from build123d import *

# Parameters (mm, degrees)
SKETCH1_W           = 25
SKETCH1_H           = 40
BOSS_EXTRUDE1_DEPTH = 8
FILLET1_R           = 2
CUT_EXTRUDE1_DEPTH  = 0.1


with BuildPart() as part:
    # Sketch1 → Boss-Extrude1 (new body)
    with BuildSketch(Plane.XY):
        Rectangle(SKETCH1_W, SKETCH1_H)
    extrude(amount=BOSS_EXTRUDE1_DEPTH)

    # Fillet1
    fillet1_edges = [part.edges().sort_by_distance(p)[0] for p in [
        (-12.5, 0, 8),
        (0, -20, 8),
        (12.5, 0, 8),
        (0, -20, 0),
        (-12.5, 0, 0),
        (0, 20, 0),
        (12.5, 0, 0),
        (12.5, -20, 4),
        (-12.5, -20, 4),
        (-12.5, 20, 4),
        (12.5, 20, 4),
        (0, 20, 8),
    ]]
    fillet(fillet1_edges, radius=FILLET1_R)

    # Sketch2 → Cut-Extrude1 (cut)
    with BuildSketch(Plane.XY.offset(8)):
        Polygon((-2.061020471, 8.237438207), (2.736573232, 8.237438207), (-0.031843364, 1.854183508), (2.068180648, 1.854183508), (-2.268382383, -6.039716385), (-0.867604628, 1.003082881), (-3.464302761, 1.003082881), align=None)
    extrude(amount=-CUT_EXTRUDE1_DEPTH, mode=Mode.SUBTRACT)


solid = part.part
Model file for the job. Use its own axes, mm. Round coordinates to 2 decimals unless told otherwise and drop trailing zeros. Loops run counter-clockwise (first coordinate to the right, second up) from the corner with the lowest first, then second, coordinate; pieces in that order, holes last. Notation, with made-up numbers: M 30,69.5 L 86,69.5 A19 cw 86,91.5 Z; hole C -27,-15.75 d1. An arc over 180 degrees is marked long. One line per question, with ' | ' between items.
1) Band-saw the part on A-A (y = 13). Give the cut face in (x, z).
Solved:
outline: M -12.5,2 A2 ccw -10.5,0 L 10.5,0 A2 ccw 12.5,2 L 12.5,6 A2 ccw 10.5,8 L -10.5,8 A2 ccw -12.5,6 Z
2) Drill centre lines: line 1 along Z through (x, y) = (1.25, 1); line 2 along Y through (x, z) = (10.5, 7); line 3 along Y through (x, z) = (6.5, 1.25). Where is each one in solid material? Low to high.
Solved:
line 1: z = 0 to 7.9 | line 2: y = -19.73 to 19.73 | line 3: y = -19.85 to 19.85
3) Band-saw the part on B-B (y = -0.5). Give the cut face in (x, z), then the cut area to 3 significant figures.
Solved:
outline: M -12.5,2 A2 ccw -10.5,0 L 10.5,0 A2 ccw 12.5,2 L 12.5,6 A2 ccw 10.5,8 L 0.77,8 L 0.77,7.9 L -1.17,7.9 L -1.17,8 L -10.5,8 A2 ccw -12.5,6 Z | area: 196 mm²
4) Mould opens along X. For faces 1 (the flat face through (0, 3, 7.9)), 2 (the flat face through (-12.5, 0, 4)), 3 (the cylindrical face through (0.15, -19.43, 7.4)) say: +X half, -X half, draft (parallel to the pull), parting line (faces both ways), or undercut.
Solved:
face 1: undercut | face 2: -X half | face 3: draft
